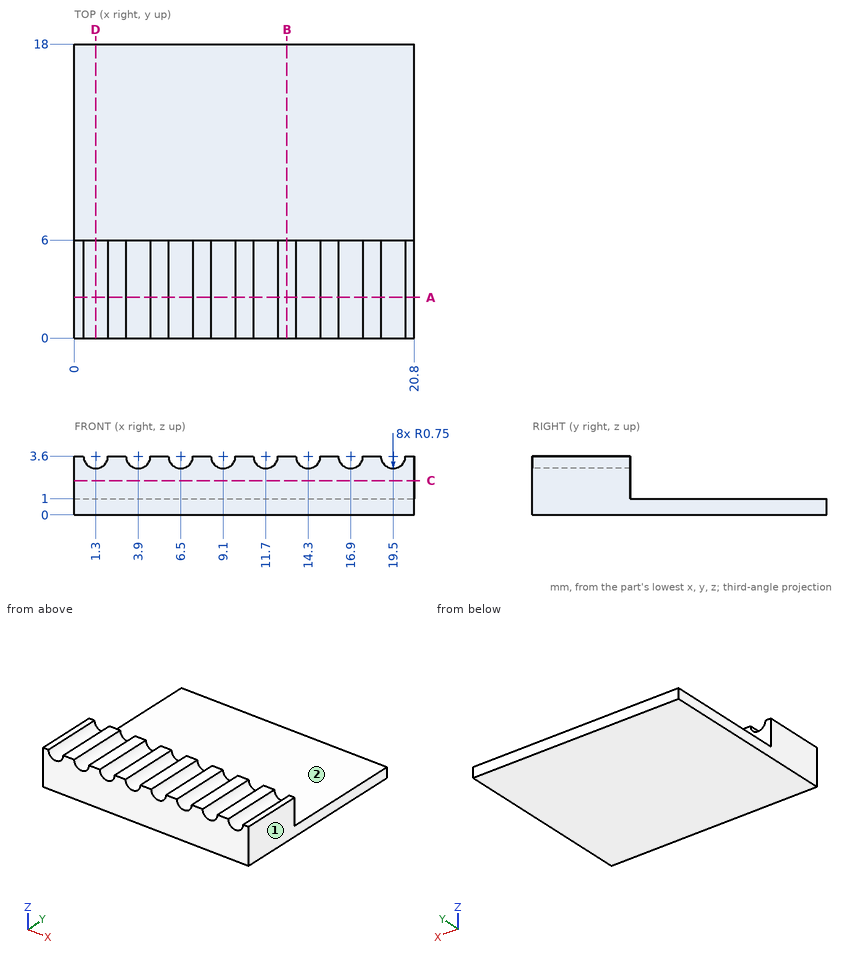
Answer from the drawing. Dimensions are ordinates in mm from the lowest x, y and z of the part. A direction names the side the tool comes from. Round coordinates to 2 decimals unless told otherwise and drop trailing zeros. Order: outer loops, then holes, each group sorted by start corner. A loop starts at its lowest first (then second) coordinate and runs counter-clockwise, first axis right, second up.
1) The part is cut by section B-B on x = 13. Write down the section's boundary in (y, z), plus the area to 3 significant figures.
2) A flat-ended cylindrical pin translates along its axis: pin 1 (1.3 mm diameter, centred on x = 12, z = 2, fed in from +Y). Find the tip coordinate at first contact, or state that the pin passes through.
3) The part is cut by section C-C on z = 2.1. Write down the section's boundary in (x, y).
4) For the marked faces 1 and 2, determine the directions among +Z, -Z, +X, -X, +Y, -Y from which every point of the face is accessible in a straight line to the end or side of a thin tool.
5) Straight lines are drawn through the part: L1, parallel to Y at x = 10.75, z = 1.3; L2, parallel to Z at x = 4.5, y = 10. For each, find the intervals that lie inside material, in ascending order.
6) The part is cut by section D-D on x = 1.3. Write down the section's boundary in (y, z).
7) The part is cut by section A-A on y = 2.5. Write down the section's boundary in (x, z), plus the area to 3 significant figures.
Resolved:
1. outline: (0, 0) - (18, 0) - (18, 1) - (6, 1) - (6, 3.6) - (0, 3.6) - close
1. area: 33.6 mm2
2. pin 1: stops at y = 6
3. outline: (0, 0) - (20.8, 0) - (20.8, 6) - (0, 6) - close
4. face 1: +Z, -Z, +X, +Y, -Y
4. face 2: +Z, +X, -X, +Y
5. L1: y = 0 to 6
5. L2: z = 0 to 1
6. outline: (0, 0) - (18, 0) - (18, 1) - (6, 1) - (6, 2.85) - (0, 2.85) - close
7. outline: (0, 0) - (20.8, 0) - (20.8, 3.6) - (20.25, 3.6) arc R0.75 cw to (18.75, 3.6) - (17.65, 3.6) arc R0.75 cw to (16.15, 3.6) - (15.05, 3.6) arc R0.75 cw to (13.55, 3.6) - (12.45, 3.6) arc R0.75 cw to (10.95, 3.6) - (9.85, 3.6) arc R0.75 cw to (8.35, 3.6) - (7.25, 3.6) arc R0.75 cw to (5.75, 3.6) - (4.65, 3.6) arc R0.75 cw to (3.15, 3.6) - (2.05, 3.6) arc R0.75 cw to (0.55, 3.6) - (0, 3.6) - close
7. area: 67.8 mm2
